Could you check a few things on this model? Use its own coordinates, in mm. Round coordinates to 2 decimals unless told otherwise and drop trailing zeros. Write each loop counter-clockwise with the first axis right and the second up, starting at its lowest first coordinate (ties: lowest second). Pieces come first, ordered by that corner, then holes. Notation, with made-up numbers: M 40.5,-35.75 L 82.5,-35.75 A12 cw 82.5,-23.75 Z; hole C 52.25,20 d9. An arc over 180 degrees is marked long. One line per question, with ' | ' between items. Start each with the question number.
```python
from build123d import *

# Parameters (mm, degrees)
SKETCH1_R           = 5
BOSS_EXTRUDE1_DEPTH = 7
FILLET2_R           = 0.2
FILLET3_R           = 0.2


with BuildPart() as part:
    # Sketch1 → Boss-Extrude1 (new body)
    with BuildSketch(Plane.XY):
        with Locations(Location((0, 0, 0), (0, 0, 180))):
            Circle(SKETCH1_R)
    extrude(amount=BOSS_EXTRUDE1_DEPTH)

    # Fillet2
    fillet2_edges = [part.edges().sort_by_distance(p)[0] for p in [
        (5, 0, 7),
    ]]
    fillet(fillet2_edges, radius=FILLET2_R)

    # Fillet3
    fillet3_edges = [part.edges().sort_by_distance(p)[0] for p in [
        (5, 0, 0),
    ]]
    fillet(fillet3_edges, radius=FILLET3_R)

    # Sketch4 → Revolve1 (revolve)
    with BuildSketch(Plane(origin=(0, 0, 0), x_dir=(1, 0, 0), z_dir=(0, 1, 0))):
        with BuildLine():
            Line((4.8, 0), (0.97819093, 3.230361511))
            ThreePointArc((0.97819093, 3.230361511), (1.18953252, 4.638794693), (0, 5.421968799))
            Line((0, 5.421968799), (0, 0))
            Line((0, 0), (4.8, 0))
        make_face()
    revolve(axis=Axis((0, 0, -5.421968799), (0, 0, 1)))


solid = part.part
```
1. I'm going to push flat-ended pins straight in: P1, Ø1.5, axis at x = -1.5, y = 3.5, coming from the -Z side; P2, Ø3, axis at x = 0.5, z = -3.5, coming from the +Y side; P3, Ø3, axis at x = -3, y = 3.5, coming from the -Z side. Where does each tip first touch, or does it pass through?
2. I need wall thicknesses on line 1 along Z through (x, y) = (2.25, 4); line 2 along Y through (x, z) = (-4.25, 6); line 3 along X through (y, z) = (-1.5, 6). Which ranges of each line are inside material? Lowest first, please. Write a range as from..to.
3. Suppose I cut it at B-B (z = -0.5). Write out the boundary of the cut face in (x, y), and give its area (3 significant figures).
4. Suppose I cut it at A-A (z = 6). Write out the boundary of the cut face in (x, y).
Computed:
1) P1: stops at z = -1.47 | P2: stops at y = 2.4 | P3: stops at z = -1.43
2) line 1: z = -0.18..7 | line 2: y = -2.63..2.63 | line 3: x = -4.77..4.77
3) outline: C 0,0 d8.42 | area: 55.6 mm²
4) outline: C 0,0 d10
